Can you work these out from the drawing? Everything is in mm from the part's minimum corner. Coordinates: 2 decimals unless noted, no trailing zeros. Order: outer loops, then holes, each group sorted by start corner. A loop starts at its lowest first (then second) coordinate and runs counter-clockwise, first axis right, second up. Notation, with made-up numbers: (42.25, 4.25) - (53.25, 4.25) arc R18 ccw to (53.25, 28.25) - close; hole circle Ø4 at (-38.5, 67.5). An arc over 180 degrees is marked (long way). Use a Markdown table: item, result. Add a question column.
(1) I want a section at D-D (x = 97). List the corners of the cut face in (y, z) for me, and give its area (3 significant figures).
(2) We'd pull the mould along X, two halves only. Please class the marked faces 1 and 2: pulls with the +X half, pulls with the -X half, needs draft (parallel to the pull), parting line crosses it, or undercut.
(3) I want a section at C-C (y = 67). List the corners of the cut face in (x, z) for me.
(4) I want a section at A-A (z = 0.85). List the corners of the cut face in (x, y) for me.
(5) I want a section at B-B (x = 59). List the corners of the cut face in (y, z) for me, and give its area (3 significant figures).
(6) If I drill on L1, parallel to Y at x = 70, z = 1.45; L2, parallel to Y at x = 38.5, z = 3.4; L3, parallel to X at y = 67.5, z = 2.1, over which ranges is the centre line in solid material (lowest first)? Write a range as [from, to].
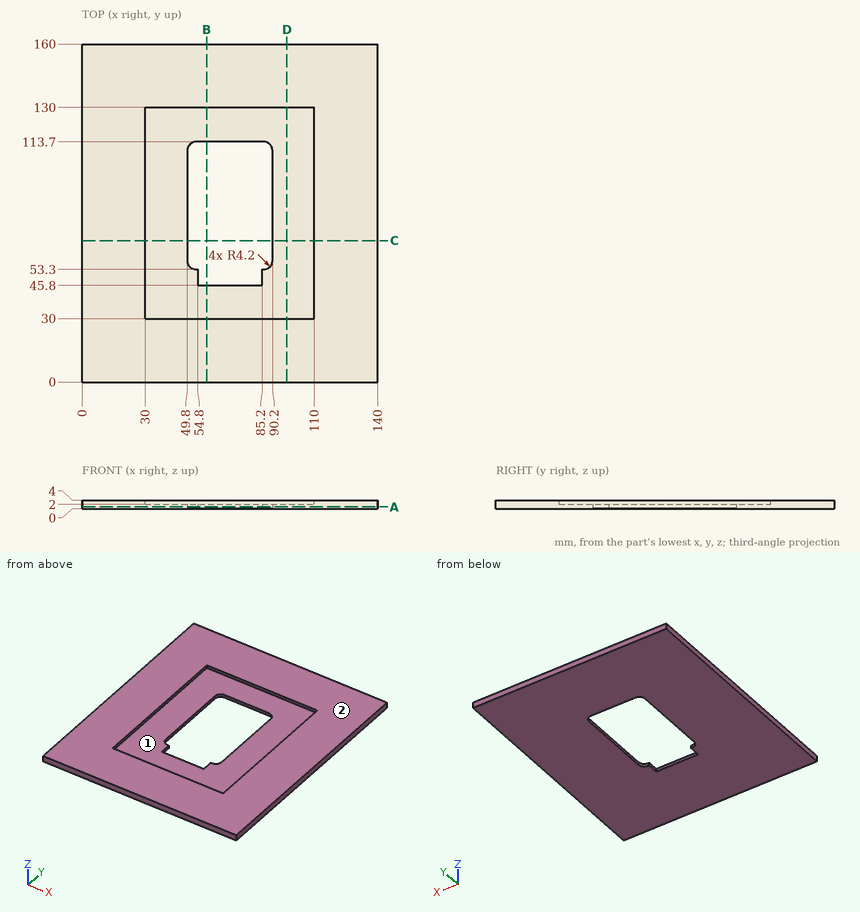
Answers follow:
| question | item | result |
|---|---|---|
| 1 | outline | (0, 0) - (160, 0) - (160, 4) - (130, 4) - (130, 2) - (30, 2) - (30, 4) - (0, 4) - close |
| 1 | area | 440 mm² |
| 2 | face 1 | undercut |
| 2 | face 2 | needs draft |
| 3 | outline | (0, 0) - (49.8, 0) - (49.8, 2) - (30, 2) - (30, 4) - (0, 4) - close; (90.2, 0) - (140, 0) - (140, 4) - (110, 4) - (110, 2) - (90.2, 2) - close |
| 4 | outline | (0, 0) - (140, 0) - (140, 160) - (0, 160) - close; hole (49.8, 57.5) arc R4.2 ccw to (54, 53.3) - (54.8, 53.3) - (54.8, 45.8) - (85.2, 45.8) - (85.2, 53.3) - (86, 53.3) arc R4.2 ccw to (90.2, 57.5) - (90.2, 109.5) arc R4.2 ccw to (86, 113.7) - (54, 113.7) arc R4.2 ccw to (49.8, 109.5) - close |
| 5 | outline | (0, 0) - (45.8, 0) - (45.8, 2) - (30, 2) - (30, 4) - (0, 4) - close; (113.7, 0) - (160, 0) - (160, 4) - (130, 4) - (130, 2) - (113.7, 2) - close |
| 5 | area | 304 mm² |
| 6 | L1 | y = [0, 45.8], [113.7, 160] |
| 6 | L2 | y = [0, 30], [130, 160] |
| 6 | L3 | x = [0, 30], [110, 140] |
